Input: part model. Units: mm. Frame: model coordinates. Face numbers are marked on the shaded views. A direction names the side the tool comes from. Round coordinates to 2 decimals unless told otherwise and drop trailing zeros. Order: outer loops, then holes, each group sorted by start corner. A loop starts at its lowest first (then second) coordinate and runs counter-clockwise, first axis right, second up. Notation, with made-up numbers: (81, 88.5) -> (140, 88.5) arc R21 ccw to (140, 94.5) -> close; hole circle Ø5 at (86, 4.5). An arc over 180 degrees is marked (long way). Use a Markdown table: item, result.
from build123d import *

# Parameters (mm, degrees)
SKETCH002_R                   = 4
SKETCH002_R_2                 = 2.1
PAD_DEPTH                     = 9.9
SKETCH002_LINEARPATTERN_2_R   = 4
SKETCH002_LINEARPATTERN_2_R_2 = 2.1
PAD_LINEARPATTERN_2_DEPTH     = 9.9
LINEARPATTERN001_COUNT        = 2
LINEARPATTERN001_PITCH        = 103


with BuildPart() as part:
    # AdditivePipe: sweep along a path in Sketch
    with BuildLine(Plane.YZ) as additivepipe_path:
        Line((-72.5, 17.5), (-72.5, 5))
        ThreePointArc((-72.5, 5), (-71.035534, 1.464466), (-67.5, 0))
        Line((-67.5, 0), (67.5, 0))
        ThreePointArc((67.5, 0), (71.035534, 1.464466), (72.5, 5))
        Line((72.5, 5), (72.5, 17.5))
    # Sketch001 → AdditivePipe (sweep)
    with BuildSketch(Plane.XY.offset(17.5)):
        Polygon((0, -72.5), (-136.1, -72.5), (-136.1, -68.9), (-134.9, -68.9), (-134.9, -71.3), (-4.9, -71.3), (-4.9, -68.9), (-3.7, -68.9), (-3.7, -71.3), (-1.2, -71.3), (-1.2, -68.9), (0, -68.9), align=None)
    sweep(path=additivepipe_path.line)

    # Sketch002 → Pad (new body)
    with BuildSketch(Plane.XY.offset(1.2)):
        with Locations((-128.9, -49.535)):
            Circle(SKETCH002_R)
        with Locations((-128.9, -49.535)):
            Circle(SKETCH002_R_2, mode=Mode.SUBTRACT)
    pad = extrude(amount=PAD_DEPTH)

    # Sketch002 LinearPattern 2 → Pad LinearPattern 2 (add)
    with BuildSketch(Plane(origin=(115, 0, 1.2), x_dir=(1, 0, 0), z_dir=(0, 0, 1))):
        with Locations((-128.9, -49.535)):
            Circle(SKETCH002_LINEARPATTERN_2_R)
        with Locations((-128.9, -49.535)):
            Circle(SKETCH002_LINEARPATTERN_2_R_2, mode=Mode.SUBTRACT)
    pad_linearpattern_2 = extrude(amount=PAD_LINEARPATTERN_2_DEPTH)

    # LinearPattern001: Pad, Pad LinearPattern 2 ×2
    with Locations(*[(0, i * LINEARPATTERN001_PITCH, 0) for i in range(1, LINEARPATTERN001_COUNT)]):
        add(pad)
        add(pad_linearpattern_2)


solid = part.part
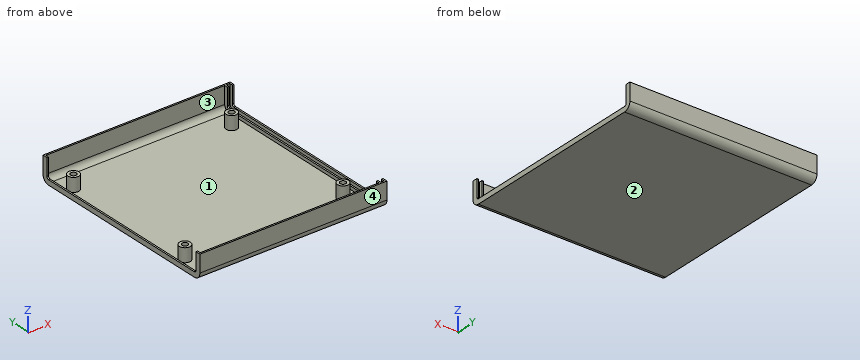
1) Set-up query: the marked faces 3 and 4. Return all of +Z, -Z, +X, -X, +Y, -Y with unobstructed straight access to the full face (end or side cutting, diameter ignored); none if empty.
Results found:
| item | result |
|---|---|
| face 3 | +Z |
| face 4 | +Z, -Z, +X, -X, -Y |
2) Cut plane A-A on z = 9.5. Count the separate pieces of the cut face and the enclosed holes in it, and give its area (3 significant figures).
Results found:
| item | result |
|---|---|
| separate pieces | 6 |
| enclosed holes | 4 |
| area | 490 mm² |
3) Cut plane B-B on x = -13.9. Return loops of the section in (y, z) (3 decimals), and give its area (3 significant figures).
Results found:
| item | result |
|---|---|
| outline | (-72.5, 5) arc R5 ccw to (-67.5, 0) -> (67.5, 0) arc R5 ccw to (72.5, 5) -> (72.5, 17.5) -> (71.3, 17.5) -> (71.3, 5) arc R3.8 cw to (67.5, 1.2) -> (57.465, 1.2) -> (57.465, 11.1) -> (55.565, 11.1) -> (55.565, 1.2) -> (51.365, 1.2) -> (51.365, 11.1) -> (49.465, 11.1) -> (49.465, 1.2) -> (-45.535, 1.2) -> (-45.535, 11.1) -> (-47.435, 11.1) -> (-47.435, 1.2) -> (-51.635, 1.2) -> (-51.635, 11.1) -> (-53.535, 11.1) -> (-53.535, 1.2) -> (-67.5, 1.2) arc R3.8 cw to (-71.3, 5) -> (-71.3, 17.5) -> (-72.5, 17.5) -> close |
| area | 284 mm² |
4) Cut plane D-D on x = -106.5. Return loops of the section in (y, z), and give its area (3 significant figures).
Results found:
| item | result |
|---|---|
| outline | (-72.5, 5) arc R5 ccw to (-67.5, 0) -> (67.5, 0) arc R5 ccw to (72.5, 5) -> (72.5, 17.5) -> (71.3, 17.5) -> (71.3, 5) arc R3.8 cw to (67.5, 1.2) -> (-67.5, 1.2) arc R3.8 cw to (-71.3, 5) -> (-71.3, 17.5) -> (-72.5, 17.5) -> close |
| area | 209 mm² |
5) Pull-direction query (X, two-part tool) for the marked faces 1 and 2; classes: +X half, -X half, draft (parallel to the pull), parting line (faces both ways), or undercut.
Results found:
| item | result |
|---|---|
| face 1 | undercut |
| face 2 | draft |
6) Pin query (flat end, axial travel): pin 1 Ø3.5 at (x, y) = (-130, -49.5) entering from +Z; pin 2 Ø1.3 at (x, y) = (-128, 54.5) entering from +Z; pin 3 Ø1 at (x, z) = (-82, 2.5) entering from +Y. Return the tip coordinate at first contact, or that it passes through.
Results found:
| item | result |
|---|---|
| pin 1 | stops at z = 11.1 |
| pin 2 | stops at z = 1.2 |
| pin 3 | stops at y = 72.08 |
7) Cut plane C-C on y = 21. Return loops of the section in (x, z).
Results found:
| item | result |
|---|---|
| outline | (-136.1, 0) -> (0, 0) -> (0, 3.6) -> (-1.2, 3.6) -> (-1.2, 1.2) -> (-3.7, 1.2) -> (-3.7, 3.6) -> (-4.9, 3.6) -> (-4.9, 1.2) -> (-134.9, 1.2) -> (-134.9, 3.6) -> (-136.1, 3.6) -> close |
8) Line query: L1, parallel to X at y = 21, z = 1.25; L2, parallel to Y at x = -111.5, z = 8; L3, parallel to Z at x = -36, y = 41. Output: solid intervals per line, ascending. Write a range as [from, to].
Results found:
| item | result |
|---|---|
| L1 | x = [-136.1, -134.9], [-4.9, -3.7], [-1.2, 0] |
| L2 | y = [-72.5, -71.3], [71.3, 72.5] |
| L3 | z = [0, 1.2] |
